Work out the finished part from the listing and answer in its coordinate system (mm). Give positions to 0.01 mm unless a question says otherwise; leave off trailing zeros. Order: outer loops, then holes, each group sorted by start corner. A loop starts at its lowest first (then second) coordinate and runs counter-clockwise, first axis right, second up. Notation, with made-up numbers: (33.5, 65) - (87.5, 65) arc R16 ccw to (87.5, 89) - close; hole circle Ø5 at (50, -36). An arc over 180 degrees is marked (long way). Put each result on its own line as item: value.
Autodesk Inventor part; units mm, degrees
ref_plane "YZ Plane" through (0, 0, 0) normal (1, 0, 0) x (0, 1, 0)
ref_plane "XZ Plane" through (0, 0, 0) normal (0, 1, 0) x (-1, 0, 0)
ref_plane "XY Plane" through (0, 0, 0) normal (0, 0, 1) x (1, 0, 0)
sketch "Sketch1" plane through (0, 0, 0) normal (0, 1, 0) x (-1, 0, 0)
  circle A0 centre (-40.7913, 50.1867) radius 2.1
  circle A1 centre (-65.133, 50.1867) radius 2.1
  line L0 (-65.3307, 56.5367) -> (-38.9924, 56.5367)
  spline S0 degree 3 poles (-76.2574, 53.0916) (-75.8034, 53.4094) (-74.4464, 54.3628) (-71.9795, 55.7143) (-68.6599, 56.5178) (-66.439, 56.5367) (-65.3307, 56.5367) knots 0 0 0 0 0.147326 0.441978 0.73663 1.031282 1.031282 1.031282 1.031282
  spline S1 degree 3 poles (-89.4746, 33.9199) (-89.4746, 34.7907) (-89.485, 37.3864) (-88.662, 41.8159) (-85.6065, 46.4828) (-82.7779, 48.5258) (-81.3513, 49.5248) knots 0 0 0 0 0.176446 0.529337 0.882228 1.235119 1.235119 1.235119 1.235119
  line L1 (-81.3513, 49.5248) -> (-76.2574, 53.0916)
  line L2 (-89.4746, 23.1867) -> (-89.4746, 33.9199)
  spline S2 degree 3 poles (-83.1246, 16.8367) (-83.5996, 16.8367) (-84.5396, 16.8415) (-85.939, 17.1545) (-87.2739, 17.9007) (-88.4105, 19.0375) (-89.1576, 20.3727) (-89.4699, 21.7718) (-89.4746, 22.7117) (-89.4746, 23.1867) knots 0 0 0 0 0.123366 0.246731 0.370097 0.493463 0.616828 0.740194 0.86356 0.86356 0.86356 0.86356
  spline S3 degree 3 poles (-76.7746, 23.1867) (-76.7746, 22.7117) (-76.7794, 21.7718) (-77.0925, 20.3724) (-77.8386, 19.0375) (-78.9754, 17.9008) (-80.3107, 17.1538) (-81.7098, 16.8415) (-82.6497, 16.8367) (-83.1246, 16.8367) knots 0 0 0 0 0.123366 0.246731 0.370097 0.493463 0.616828 0.740194 0.86356 0.86356 0.86356 0.86356
  circle A2 centre (-83.1246, 23.1867) radius 2.3114
  circle A3 centre (-83.1246, 35.8867) radius 2.3114
  spline S4 degree 3 poles (-74.0669, 38.4483) (-74.5424, 38.1153) (-75.4851, 37.433) (-76.5038, 35.8783) (-76.7782, 34.4018) (-76.7746, 33.537) (-76.7746, 33.2467) knots 0 0 0 0 0.11763 0.235261 0.352891 0.411706 0.411706 0.411706 0.411706
  line L3 (-76.7746, 33.2467) -> (-76.7746, 23.1867)
  line L4 (-68.0115, 42.6883) -> (-74.0669, 38.4483)
  spline S5 degree 3 poles (-64.3693, 43.8367) (-64.7387, 43.8367) (-65.4747, 43.8285) (-66.7721, 43.5188) (-67.5576, 43.0062) (-68.0115, 42.6883) knots 0 0 0 0 0.098217 0.196435 0.343761 0.343761 0.343761 0.343761
  line L5 (-41.555, 43.8367) -> (-64.3693, 43.8367)
  spline S6 degree 3 poles (-37.9128, 42.6883) (-38.2154, 42.9002) (-38.823, 43.3156) (-40.0634, 43.806) (-41.0009, 43.8367) (-41.555, 43.8367) knots 0 0 0 0 0.098217 0.196435 0.343761 0.343761 0.343761 0.343761
  line L6 (-31.8574, 38.4483) -> (-37.9128, 42.6883)
  line L7 (-29.1496, 10.4867) -> (-29.1496, 33.2467)
  spline S7 degree 3 poles (-29.1496, 33.2467) (-29.1496, 33.8272) (-29.1679, 34.9915) (-29.8568, 36.7161) (-30.9093, 37.7887) (-31.6197, 38.2818) (-31.8574, 38.4483) knots 0 0 0 0 0.11763 0.235261 0.352891 0.411706 0.411706 0.411706 0.411706
  line L8 (-35.0553, 55.911) -> (3.1371, 43.4575)
  arc A4 (-35.0553, 55.911) -> (-38.9924, 56.5367) centre (-38.9924, 43.8367) ccw
  circle A5 centre (90.9711, -52.3822) radius 2.1844
  circle A6 centre (-22.7996, 35.8867) radius 2.1844
  circle A7 centre (1.1686, 37.4204) radius 2.0955
  arc A8 (5.9122, 33.199) -> (3.1371, 43.4575) centre (1.1686, 37.4204) ccw
  circle A9 centre (-22.7996, 10.4867) radius 2.1971
  arc A10 (-29.1496, 10.4867) -> (-18.056, 6.2653) centre (-22.7996, 10.4867) ccw
  line L9 (-18.056, 6.2653) -> (5.9122, 33.199)
  point P0 (0, 0)
  point P1 (99.9514, -43.4019)
  point P2 (97.0418, -61.7217)
  dimension "d8" = 12.7
  dimension "d9" = 12.7
extrude "Extrusion1" add sketch "Sketch1" along normal blind 1.5875 contours L0 A4 L8 A8 L9 A10 L7 S7 L6 S6 L5 S5 L4 S4 L3 S3 S2 L2 S1 L1 S0
properties part number "funnel_gusset_full" material "Acetal Resin, Black"
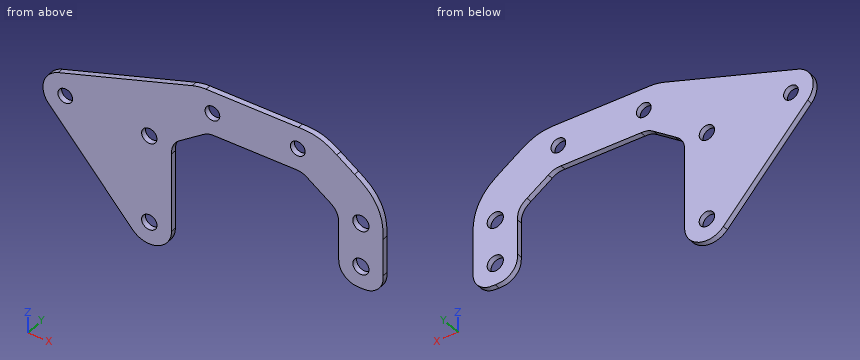
(1) Section D-D, the plane x = 36.5 is taken. Write down the section's boundary in (y, z).
Geometry check:
outline: (0, 41.7) - (1.59, 41.7) - (1.59, 56.29) - (0, 56.29) - close
(2) Section B-B, the plane x = 54.5 is taken. Write down the section's boundary in (y, z).
Geometry check:
outline: (0, 43.84) - (1.59, 43.84) - (1.59, 56.54) - (0, 56.54) - close
(3) Section A-A, the plane z = 24.5 is taken. Write down the section's boundary in (x, y).
Geometry check:
outline: (1.83, 0) - (29.15, 0) - (29.15, 1.59) - (1.83, 1.59) - close; (76.77, 0) - (81.22, 0) - (81.22, 1.59) - (76.77, 1.59) - close; (85.03, 0) - (89.47, 0) - (89.47, 1.59) - (85.03, 1.59) - close
(4) Given pin 1 (2.5 mm diameter, centred on x = 40.79, z = 50.19, fed in from +Y); pin 2 (0.8 mm diameter, centred on y = 1, z = 30.5, fed in from -X), each flat-ended and moving along its own axis, determine where each tip first touches the part or whether it passes through.
Geometry check:
pin 1: passes through
pin 2: stops at x = -3.87
(5) Section C-C, the plane y = 0.4 is taken. Count the separate pieces of the cut face and the enclosed holes in it, then the cut area to 3 significant figures.
Geometry check:
separate pieces: 1
enclosed holes: 7
area: 2,100 mm²
(6) Straight lines are drawn through the part: line 1 (Z direction, x = 21, y = 0.4); line 2 (Z direction, x = 82, y = 0.75); line 3 (X direction, y = 1, z = 23). For each, find the intervals that lie inside material, in ascending order.
Geometry check:
line 1: z = 4.4 to 9.23, 11.75 to 34.65, 37.12 to 51.33
line 2: z = 16.87 to 21.17, 25.21 to 33.87, 37.91 to 49.07
line 3: x = 3.16 to 29.15, 76.77 to 80.82, 85.43 to 89.47
